```python
from build123d import *

# Parameters (mm, degrees)
ESQUISSE2_R                  = 2
ENL_V_MAT_EXTRU_1_DEPTH      = 17
CONG_1_R                     = 0.5
ENL_V_MAT_EXTRU_2_DEPTH      = 8
R_P_TITION_CIRCULAIRE1_COUNT = 10
ESQUISSE4_W                  = 1.25
ESQUISSE4_H                  = 5


with BuildPart() as part:
    # Esquisse1 → Révolution1 (revolve)
    with BuildSketch(Plane.XY):
        Polygon((0, 0), (0, 3.725), (8, 3.725), (8, 5), (16, 5), (16, 0), align=None)
    revolve(axis=Axis((16, 0, 0), (-1, 0, 0)))

    # Esquisse2 → Enlèv. mat.-Extru.1 (cut, through all)
    with BuildSketch(Plane(origin=(16, 0, 0), x_dir=(0, 0, -1), z_dir=(1, 0, 0))):
        with Locations(Location((0, 0, 0), (0, 0, 90))):  # turned: the seam where the file's is
            Circle(ESQUISSE2_R)
    extrude(amount=-ENL_V_MAT_EXTRU_1_DEPTH, mode=Mode.SUBTRACT)

    # Congé1
    cong_1_edges = [part.edges().sort_by_distance(p)[0] for p in [
        (8, -5, 0),
    ]]
    fillet(cong_1_edges, radius=CONG_1_R)

    # Esquisse3 → Enlèv. mat.-Extru.2 (cut)
    with BuildSketch(Plane.ZY):
        Polygon((0.675560046, 3.69719402), (0.56250399, 2.89275838), (1.245245427, 2.67092224), (1.626616562, 3.388177026), align=None)
    enl_v_mat_extru_2 = extrude(amount=-ENL_V_MAT_EXTRU_2_DEPTH, mode=Mode.SUBTRACT)

    # Répétition circulaire1: Enlèv. mat.-Extru.2 ×10 about axis
    r_p_tition_circulaire1_axis = Axis((0, 0, 0), (1, 0, 0))
    for i in range(1, R_P_TITION_CIRCULAIRE1_COUNT):
        add(enl_v_mat_extru_2.rotate(r_p_tition_circulaire1_axis, i * 360 / R_P_TITION_CIRCULAIRE1_COUNT), mode=Mode.SUBTRACT)

    # Esquisse4 → Trou taraudé M31 (revolve, cut)
    with BuildSketch(Plane(origin=(13, 0, 0), x_dir=(0, 0, -1), z_dir=(1, 0, 0))):
        with Locations((0.625, 2.5)):
            Rectangle(ESQUISSE4_W, ESQUISSE4_H)
    revolve(axis=Axis((13, -6.35, 0), (0, 1, 0)), mode=Mode.SUBTRACT)


solid = part.part
```
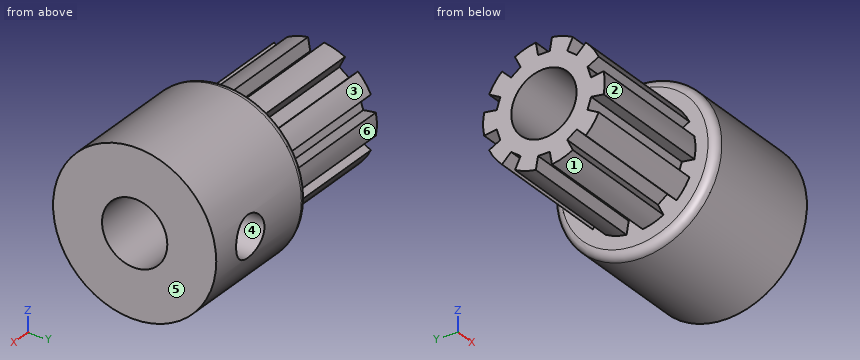
Design review of the part built by this model. Coordinates are the model's own, in mm. Face numbers are marked on the shaded views. A direction names the side the tool comes from. Give positions to 0.01 mm unless a question says otherwise; leave off trailing zeros. Order: outer loops, then holes, each group sorted by start corner. A loop starts at its lowest first (then second) coordinate and runs counter-clockwise, first axis right, second up. Notation, with made-up numbers: M 7,55.25 L 14,55.25 A28 ccw 14,79.25 Z; hole C 28,76 d10. An arc over 180 degrees is marked long. One line per question, with ' | ' between items. Start each with the question number.
Q1. We need section C-C (x = 13.75). Write out the cut boundary in (y, z).
Q2. We need section A-A (z = 0). Write out the cut boundary in (x, y) (3 decimals), plus the area to 3 significant figures.
Q3. We need section B-B (y = 0). Write out the cut boundary in (x, z) (3 decimals).
Q4. Machinability: for the marked faces 1, 2 and 3, which of the approach directions +Z, -Z, +X, -X, +Y, -Y give a long, thin tool a straight path to every point of the face, cutting with its end or side? Answer none if there is none.
Q5. The part is to be moulded in two halves that separate along X. For the marked faces 4, 5 and 6, say which applies: +X half, -X half, draft (parallel to the pull), parting line (faces both ways), or undercut.
Q6. For pin 1 Ø1 at (x, z) = (6, 2.5) entering from +Y; pin 2 Ø3 at (x, y) = (13.5, -2.5) entering from -Z; pin 3 Ø0.6 at (x, y) = (4, 0) entering from -Z (3 decimals), all flat-tipped, find the tip position at first contact; note any pin that passes through.
Q7. For L1, parallel to Z at x = 10.25, y = 0; L2, parallel to X at y = 2.9, z = 0; L3, parallel to Z at x = 3.75, y = 0 (3 decimals), list the stretches that pass through material, from the lowest coordinate up. Write a range as [from, to].
Returned:
1) outline: M 1.73,-1 A2 cw long 1.73,1 L 4.9,1 A5 ccw long 4.9,-1 Z
2) outline: M 0,-3.725 L 8,-3.725 L 8,-4.5 A0.5 ccw 8.5,-5 L 16,-5 L 16,-2 L 0,-2 Z; M 0,2 L 11.75,2 L 11.75,5 L 8.5,5 A0.5 ccw 8,4.5 L 8,3.725 L 0,3.725 Z; M 14.25,2 L 16,2 L 16,5 L 14.25,5 Z | area: 68.0 mm2
3) outline: M 0,-2.925 L 8,-2.925 L 8,-4.5 A0.5 ccw 8.5,-5 L 16,-5 L 16,-2 L 0,-2 Z; M 0,2 L 16,2 L 16,5 L 8.5,5 A0.5 ccw 8,4.5 L 8,2.925 L 0,2.925 Z
4) face 1: -Z, -X, -Y | face 2: -X, -Y | face 3: +Z, -X, +Y
5) face 4: undercut | face 5: +X half | face 6: draft
6) pin 1: y = 3.14 | pin 2: z = -4.9 | pin 3: z = -2.925
7) L1: [-5, -2], [2, 5] | L2: [0, 11.75], [14.25, 16] | L3: [-2.925, -2], [2, 2.925]
